```python
from build123d import *

# Parameters (mm, degrees)
SKICA1_W                 = 85
SKICA1_H                 = 17.5
SKICA1_R                 = 3.05
P_IDAT_VYSUNUT_M1_DEPTH  = 3
SKICA3_W                 = 65
SKICA3_H                 = 40
P_IDAT_VYSUNUT_M2_DEPTH  = 17.5
ZAOBLIT2_R               = 17
SKICA4_R                 = 6
SKICA4_R_2               = 4.1
P_IDAT_VYSUNUT_M3_DEPTH  = 3
SKICA4_2_R               = 4.1
ODEBRAT_VYSUNUT_M1_DEPTH = 4
SKICA5_W                 = 20
SKICA5_H                 = 18
ODEBRAT_VYSUNUT_M2_DEPTH = 63.940448044
SKICA7_R                 = 3.25
ODEBRAT_VYSUNUT_M4_DEPTH = 50
SKICA8_W                 = 35
SKICA8_H                 = 21
SKICA8_R                 = 3.05
P_IDAT_VYSUNUT_M4_DEPTH  = 3
ZAOBLIT1_R               = 4
EBRO4_REACH              = 69.382
SKICA12_WALL_W           = 158.350715196
SKICA12_WALL_H           = 10


with BuildPart() as part:
    # Skica1 → P_idat vysunut_m1 (new body)
    with BuildSketch(Plane(origin=(0, 0, 0), x_dir=(1, 0, 0), z_dir=(0, 1, 0))):
        Rectangle(SKICA1_W, SKICA1_H)
        with Locations(Location((-37.5, 0, 0), (0, 0, 270))):
            Circle(SKICA1_R, mode=Mode.SUBTRACT)
        with Locations(Location((37.5, 0, 0), (0, 0, 270))):
            Circle(SKICA1_R, mode=Mode.SUBTRACT)
    extrude(amount=P_IDAT_VYSUNUT_M1_DEPTH)

    # Skica3 → P_idat vysunut_m2 (add)
    with BuildSketch(Plane.XY.offset(8.75)):
        with Locations((0, 23)):
            Rectangle(SKICA3_W, SKICA3_H)
    extrude(amount=-P_IDAT_VYSUNUT_M2_DEPTH)

    # Zaoblit2
    zaoblit2_edges = [part.edges().sort_by_distance(p)[0] for p in [
        (32.5, 43, 0),
        (-32.5, 43, 0),
    ]]
    fillet(zaoblit2_edges, radius=ZAOBLIT2_R)

    # Skica4 → P_idat vysunut_m3 (add)
    with BuildSketch(Plane.XY.offset(8.75)):
        with Locations(Location((-20, 27, 0), (0, 0, 180))):
            Circle(SKICA4_R)
        with Locations((-20, 27)):
            Circle(SKICA4_R_2, mode=Mode.SUBTRACT)
        with Locations(Location((20, 27, 0), (0, 0, 180))):
            Circle(SKICA4_R)
        with Locations((20, 27)):
            Circle(SKICA4_R_2, mode=Mode.SUBTRACT)
    extrude(amount=P_IDAT_VYSUNUT_M3_DEPTH)

    # Skica4_2 → Odebrat vysunut_m1 (cut)
    with BuildSketch(Plane.XY.offset(8.75)):
        with Locations((20, 27)):
            Circle(SKICA4_2_R)
        with Locations((-20, 27)):
            Circle(SKICA4_2_R)
    extrude(amount=-ODEBRAT_VYSUNUT_M1_DEPTH, mode=Mode.SUBTRACT)

    # Skica5 → Odebrat vysunut_m2 (cut, through all)
    with BuildSketch(Plane.XY.offset(8.75)):
        with Locations((0, 22)):
            Rectangle(SKICA5_W, SKICA5_H)
    extrude(amount=-ODEBRAT_VYSUNUT_M2_DEPTH, mode=Mode.SUBTRACT)

    # Skica7 → Odebrat vysunut_m4 (cut)
    with BuildSketch(Plane(origin=(32.5, 0, 0), x_dir=(0, 0, -1), z_dir=(1, 0, 0))):
        with Locations(Location((1.25, 22, 0), (0, 0, 90))):
            Circle(SKICA7_R)
    extrude(amount=-ODEBRAT_VYSUNUT_M4_DEPTH, mode=Mode.SUBTRACT)

    # Skica8 → P_idat vysunut_m4 (add)
    with BuildSketch(Plane.XZ):
        with Locations((0, 19.25)):
            Rectangle(SKICA8_W, SKICA8_H)
        with Locations(Location((-12.5, 25, 0), (0, 0, 270))):
            Circle(SKICA8_R, mode=Mode.SUBTRACT)
        with Locations(Location((12.5, 25, 0), (0, 0, 90))):
            Circle(SKICA8_R, mode=Mode.SUBTRACT)
    extrude(amount=-P_IDAT_VYSUNUT_M4_DEPTH)

    # Zaoblit1
    zaoblit1_edges = [part.edges().sort_by_distance(p)[0] for p in [
        (42.5, 1.5, 8.75),
        (-42.5, 1.5, 8.75),
        (-42.5, 1.5, -8.75),
        (42.5, 1.5, -8.75),
        (17.5, 1.5, 8.75),
        (-17.5, 1.5, 8.75),
        (-17.5, 1.5, 29.75),
        (17.5, 1.5, 29.75),
    ]]
    fillet(zaoblit1_edges, radius=ZAOBLIT1_R)

    # Skica12 wall → ebro4 (add, up to next)
    with BuildSketch(Plane(origin=(0, 5.5, 19.25), x_dir=(0, 0.231620527306, -0.972806214685), z_dir=(0, 0.972806214685, 0.231620527306)), mode=Mode.PRIVATE) as ebro4_sk1:
        Rectangle(SKICA12_WALL_W, SKICA12_WALL_H)
    ebro4_tool1 = extrude(ebro4_sk1.sketch, amount=-EBRO4_REACH, mode=Mode.PRIVATE) - part.part
    add(ebro4_tool1.solids().sort_by_distance((0, 5.5, 19.25))[0])


solid = part.part
```
Input: part model. Units: mm. Frame: model coordinates. A direction names the side the tool comes from. Coordinates: 2 decimals unless noted, no trailing zeros. Order: outer loops, then holes, each group sorted by start corner. A loop starts at its lowest first (then second) coordinate and runs counter-clockwise, first axis right, second up. Notation, with made-up numbers: (20.5, 51) - (42.5, 51) arc R13 ccw to (42.5, 68) - close; hole circle Ø7 at (67, 56). An arc over 180 degrees is marked (long way). Return JSON: item names as keys, results as strings.
Q1. First-contact query: pin 1 (13 mm diameter, centred on x = 22, y = 25.5, fed in from +Z); pin 2 (5 mm diameter, centred on y = 22, z = -1.25, fed in from +X); pin 3 (2 mm diameter, centred on y = 28.5, z = 4.5, fed in from -X); pin 4 (6 mm diameter, centred on x = -7.5, z = -2, fed in from -Y). Flat tips, straight axial feed; report the tip coordinate or a pass-through.
The answers:
{"pin 1": "stops at z = 11.75", "pin 2": "stops at x = -17.5", "pin 3": "stops at x = -32.43", "pin 4": "stops at y = 0"}
Q2. Cut plane A-A (x = 12.5). Return loops of the section in (y, z), then the cut area to 3 significant figures.
The answers:
{"outline": "(0, -8.75) - (43, -8.75) - (43, 8.75) - (3, 8.75) - (3, 21.95) - (0, 21.95) - close; (0, 28.05) - (3, 28.05) - (3, 29.75) - (0, 29.75) - close; hole circle Ø6.5 at (22, -1.25)", "area": "764 mm2"}
Q3. Draft query along X for faces 5 (the flat face through (32.5, 14, 0)), 6 (the flat face through (11, 3, 19)), 7 (the cylindrical face through (16.746, 24.505, 8.201)), 8 (the cylindrical face through (-16.359, 1.521, 28.547)). Return one class per face: +X half, -X half, draft (parallel to the pull), parting line (faces both ways), or undercut.
The answers:
{"face 5": "+X half", "face 6": "draft", "face 7": "undercut", "face 8": "-X half"}
Q4. Ray query, probe 1 along X at (y, z) = (15, 0.5); probe 2 along X at (y, z) = (1, 0); probe 3 along Y at (x, z) = (-4, -5.5). Return the intervals inside material, ascending.
The answers:
{"probe 1": "x = -32.5 to -10, 10 to 32.5", "probe 2": "x = -42.5 to -40.55, -34.45 to 34.45, 40.55 to 42.5", "probe 3": "y = 0 to 13, 31 to 43"}
Q5. Cut plane B-B (z = 24.5). Return loops of the section in (x, y).
The answers:
{"outline": "(-17.5, 0) - (-15.51, 0) - (-15.51, 3) - (-17.5, 3) - close; (-9.49, 0) - (9.49, 0) - (9.49, 3) - (5, 3) - (5, 4.25) - (-5, 4.25) - (-5, 3) - (-9.49, 3) - close; (15.51, 0) - (17.5, 0) - (17.5, 3) - (15.51, 3) - close"}
Q6. Access query for faces 1 (the flat face through (35, 3, -2)), 2 (the flat face through (-17.5, 1, 19)), 3 (the flat face through (-5, 4, 17)), 4 (the flat face through (17, 31, 11.75)). Directions: +Z, -Z, +X, -X, +Y, -Y. A direction counts if a zero-diameter tool reaches every point of the face in a straight line with its end or side. Return the directions, or none.
The answers:
{"face 1": "+Z, -Z, +X, +Y", "face 2": "+Z, -X, +Y, -Y", "face 3": "+Z, -X, +Y", "face 4": "+Z, +X, -X, +Y"}
Q7. Cut plane C-C (y = 7). Return loops of the section in (x, z), then the cut area to 3 significant figures.
The answers:
{"outline": "(-32.5, -8.75) - (32.5, -8.75) - (32.5, 8.75) - (5, 8.75) - (5, 12.95) - (-5, 12.95) - (-5, 8.75) - (-32.5, 8.75) - close", "area": "1,180 mm2"}
Q8. Cut plane D-D (y = 27). Return loops of the section in (x, z).
The answers:
{"outline": "(-32.47, -8.75) - (-10, -8.75) - (-10, 8.75) - (-14, 8.75) - (-14, 11.75) - (-15.9, 11.75) - (-15.9, 4.75) - (-24.1, 4.75) - (-24.1, 11.75) - (-26, 11.75) - (-26, 8.75) - (-32.47, 8.75) - close; (10, -8.75) - (32.47, -8.75) - (32.47, 8.75) - (26, 8.75) - (26, 11.75) - (24.1, 11.75) - (24.1, 4.75) - (15.9, 4.75) - (15.9, 11.75) - (14, 11.75) - (14, 8.75) - (10, 8.75) - close"}
